The model under review builds one solid part; all positions refer to its coordinate system, in mm. A direction names the side the tool comes from. Round coordinates to 2 decimals unless told otherwise and drop trailing zeros. Order: outer loops, then holes, each group sorted by start corner. A loop starts at its lowest first (then second) coordinate and runs counter-clockwise, first axis right, second up.
```python
from build123d import *

# Parameters (mm, degrees)
SKETCH2_R          = 1.2446
CUT_EXTRUDE1_DEPTH = 15.16
SKETCH4_R          = 2.5
CUT_EXTRUDE3_DEPTH = 6
CHAMFER1_SIZE      = 0.75


with BuildPart() as part:
    # Sketch1 → Revolve1 (revolve)
    with BuildSketch(Plane.XY):
        Polygon((0, 14.16), (0, 0), (7.9375, 0), (7.9375, 4.76), (6, 4.76), (6, 9.4), (7.9375, 9.4), (7.9375, 14.16), align=None)
    revolve(axis=Axis((0, 14.16, 0), (0, -1, 0)))

    # Sketch2 → Cut-Extrude1 (cut, through all)
    with BuildSketch(Plane(origin=(0, 14.16, 0), x_dir=(1, 0, 0), z_dir=(0, 1, 0))):
        Circle(SKETCH2_R)
    extrude(amount=-CUT_EXTRUDE1_DEPTH, mode=Mode.SUBTRACT)

    # Sketch4 → Cut-Extrude3 (cut)
    with BuildSketch(Plane.XZ):
        Circle(SKETCH4_R)
    extrude(amount=-CUT_EXTRUDE3_DEPTH, mode=Mode.SUBTRACT)

    # Chamfer1
    chamfer1_edges = [part.edges().sort_by_distance(p)[0] for p in [
        (-1.2446, 14.16, 0),
        (-7.9375, 14.16, 0),
        (-7.9375, 0, 0),
    ]]
    chamfer(chamfer1_edges, length=CHAMFER1_SIZE)


solid = part.part
```
(1) Insertion check: pin 1 (5 mm diameter, centred on x = -5.5, z = 4.5, fed in from -Y); pin 2 (5 mm diameter, centred on y = 10.5, z = -5.5, fed in from +X); pin 3 (2 mm diameter, centred on y = 2, z = 5.5, fed in from -X). Each pin has a flat end and moves straight along its axis. Give the tip position at first contact, or say it passes through.
Data:
pin 1: stops at y = 0
pin 2: stops at x = 7.35
pin 3: stops at x = -6.54
(2) Consider section A-A (z = 0). Write out the cut boundary in (x, y), and give its area (3 significant figures).
Data:
outline: (-7.94, 0.75) - (-7.19, 0) - (-2.5, 0) - (-2.5, 6) - (-1.24, 6) - (-1.24, 13.41) - (-1.99, 14.16) - (-7.19, 14.16) - (-7.94, 13.41) - (-7.94, 9.4) - (-6, 9.4) - (-6, 4.76) - (-7.94, 4.76) - close; (1.24, 6) - (2.5, 6) - (2.5, 0) - (7.19, 0) - (7.94, 0.75) - (7.94, 4.76) - (6, 4.76) - (6, 9.4) - (7.94, 9.4) - (7.94, 13.41) - (7.19, 14.16) - (1.99, 14.16) - (1.24, 13.41) - close
area: 155 mm2
(3) For faces 4 (the flat face through (-3, 0, 0)), 5 (the flat face through (2, 9.4, 6)), 6 (the flat face through (-1, 6, -1)), list the 3-axis set-ups (+Z, -Z, +X, -X, +Y, -Y) from which the entire face can be reached by the end or side of a thin tool; tool diameter is ignored.
Data:
face 4: +Z, -Z, +X, -X, -Y
face 5: none
face 6: -Y
(4) To check wall thickness, follow probe 1 along Z at (x, y) = (0, 8.75); probe 2 along Z at (x, y) = (0, 10.5); probe 3 along Y at (x, z) = (0.75, -6.75). State the ranges of each line that lie inside material, in increasing order.
Data:
probe 1: z = -6 to -1.24, 1.24 to 6
probe 2: z = -7.94 to -1.24, 1.24 to 7.94
probe 3: y = 0 to 4.76, 9.4 to 14.16
(5) Draft analysis for pull direction Z (two halves, no side actions). For faces 1 (the cylindrical face through (-6, 7, 0)), 2 (the cylindrical face through (-0.54, 2.96, -2.44)), 3 (the flat face through (-2, 4.76, 6)), state which applies: pulls with the +Z half, pulls with the -Z half, needs draft (parallel to the pull), parting line crosses it, or undercut.
Data:
face 1: parting line crosses it
face 2: undercut
face 3: needs draft
(6) Consider section D-D (y = 1). Write out the cut boundary in (x, z) (1 decimal), and give its area (3 significant figures).
Data:
outline: circle Ø15.9 at (0, 0); hole circle Ø5 at (0, 0)
area: 178 mm2
(7) Consider section B-B (x = 0). Write out the cut boundary in (y, z).
Data:
outline: (0, -7.19) - (0.75, -7.94) - (4.76, -7.94) - (4.76, -6) - (9.4, -6) - (9.4, -7.94) - (13.41, -7.94) - (14.16, -7.19) - (14.16, -1.99) - (13.41, -1.24) - (6, -1.24) - (6, -2.5) - (0, -2.5) - close; (0, 2.5) - (6, 2.5) - (6, 1.24) - (13.41, 1.24) - (14.16, 1.99) - (14.16, 7.19) - (13.41, 7.94) - (9.4, 7.94) - (9.4, 6) - (4.76, 6) - (4.76, 7.94) - (0.75, 7.94) - (0, 7.19) - close
(8) Consider section C-C (y = 12.5). Write out the cut boundary in (x, z) (1 decimal), and give its area (3 significant figures).
Data:
outline: circle Ø15.9 at (0, 0); hole circle Ø2.5 at (0, 0)
area: 193 mm2
